```python
from build123d import *
from build123d.topology import SkipClean

# Parameters (mm, degrees)
SKETCH_2_R          = 2
SKETCH_2_R_2        = 11
SKETCH_2_R_3        = 3
SKETCH_2_R_4        = 1.6
EXTRUDE_1_DEPTH     = 10
CUT_EXTRUDE_2_DEPTH = 4


with BuildPart() as part:
    # Эскиз2 → Бобышка-Вытянуть1 (new body)
    with BuildSketch(Plane.XY):
        with BuildLine():
            Line((-25.5006943, 139.9), (-25.5006943, 109.05))
            Line((-25.5006943, 109.05), (-25.5006943, 75.100000001))
            Line((-25.5006943, 75.100000001), (-35.4993057, 75.066643523))
            Line((-35.4993057, 75.066643523), (-35.4993057, 65.066643523))
            Line((-35.4993057, 65.066643523), (-25.5006943, 64.9))
            Line((-25.5006943, 64.9), (-25.5006943, -64.899999999))
            Line((-25.5006943, -64.899999999), (-35.4993057, -64.933356477))
            Line((-35.4993057, -64.933356477), (-35.4993057, -74.933356477))
            Line((-35.4993057, -74.933356477), (-25.5006943, -75.1))
            Line((-25.5006943, -75.1), (-25.5006943, -105.95))
            Line((-25.5006943, -105.95), (-25.5006943, -139.899999999))
            Line((-25.5006943, -139.899999999), (-35.4993057, -139.933356477))
            Line((-35.4993057, -139.933356477), (-35.4993057, -149.933356477))
            Line((-35.4993057, -149.933356477), (-25.5006943, -150.1))
            Line((-25.5006943, -150.1), (-25.5006943, -173.45))
            Line((-25.5006943, -173.45), (-25.5006943, -199.899999999))
            Line((-25.5006943, -199.899999999), (-35.4993057, -199.933356477))
            Line((-35.4993057, -199.933356477), (-35.4993057, -209.933356477))
            Line((-35.4993057, -209.933356477), (-25.5006943, -210.1))
            Line((-25.5006943, -210.1), (-25.5006943, -221))
            Line((-25.5006943, -221), (-17.5006943, -229))
            Line((-17.5006943, -229), (-2.1006943, -229))
            Line((-2.1006943, -229), (-2.067337824, -238.9986114))
            Line((-2.067337824, -238.9986114), (7.932662176, -238.9986114))
            Line((7.932662176, -238.9986114), (8.099305701, -229))
            Line((8.099305701, -229), (35.4993057, -229))
            Line((35.4993057, -229), (35.4993057, -209))
            Line((35.4993057, -209), (33.4993057, -209))
            Line((33.4993057, -209), (33.4993057, -151))
            ThreePointArc((33.4993057, -151), (22.78974844, -0.441666666), (33.4993057, 150.116666668))
            Line((33.4993057, 150.116666668), (33.4993057, 208.116666668))
            Line((33.4993057, 208.116666668), (35.4993057, 208.116666668))
            Line((35.4993057, 208.116666668), (35.4993057, 229))
            Line((35.4993057, 229), (8.099305701, 229))
            Line((8.099305701, 229), (7.932662176, 238.9986114))
            Line((7.932662176, 238.9986114), (-2.067337824, 238.9986114))
            Line((-2.067337824, 238.9986114), (-2.1006943, 229))
            Line((-2.1006943, 229), (-17.5006943, 229))
            Line((-17.5006943, 229), (-25.5006943, 221))
            Line((-25.5006943, 221), (-25.5006943, 210.100000001))
            Line((-25.5006943, 210.100000001), (-35.4993057, 210.066643523))
            Line((-35.4993057, 210.066643523), (-35.4993057, 200.066643523))
            Line((-35.4993057, 200.066643523), (-25.5006943, 199.9))
            Line((-25.5006943, 199.9), (-25.5006943, 176.55))
            Line((-25.5006943, 176.55), (-25.5006943, 150.100000001))
            Line((-25.5006943, 150.100000001), (-35.4993057, 150.066643523))
            Line((-35.4993057, 150.066643523), (-35.4993057, 140.066643523))
            Line((-35.4993057, 140.066643523), (-25.5006943, 139.9))
        make_face()
        with Locations((-18.0006943, -190.5)):
            Circle(SKETCH_2_R, mode=Mode.SUBTRACT)
        with Locations((-18.0006943, -221.5)):
            Circle(SKETCH_2_R, mode=Mode.SUBTRACT)
        with Locations((-18.0006943, 190.5)):
            Circle(SKETCH_2_R, mode=Mode.SUBTRACT)
        with Locations((12.9993057, 221.5)):
            Circle(SKETCH_2_R, mode=Mode.SUBTRACT)
        with Locations((-2.5006943, -206)):
            Circle(SKETCH_2_R_2, mode=Mode.SUBTRACT)
        with Locations((-2.5006943, 206)):
            Circle(SKETCH_2_R_2, mode=Mode.SUBTRACT)
        with Locations((-18.0006943, 221.5)):
            Circle(SKETCH_2_R, mode=Mode.SUBTRACT)
        with Locations((12.9993057, -221.5)):
            Circle(SKETCH_2_R, mode=Mode.SUBTRACT)
        with Locations((12.9993057, -190.5)):
            Circle(SKETCH_2_R, mode=Mode.SUBTRACT)
        with Locations((12.9993057, 190.5)):
            Circle(SKETCH_2_R, mode=Mode.SUBTRACT)
        with Locations((-5.6006943, -153.2)):
            Circle(SKETCH_2_R_3, mode=Mode.SUBTRACT)
        with Locations((-5.6006943, 153.2)):
            Circle(SKETCH_2_R_3, mode=Mode.SUBTRACT)
        with Locations((9.4993057, -139.899999999)):
            Circle(SKETCH_2_R_4, mode=Mode.SUBTRACT)
        with Locations((9.4993057, 139.9)):
            Circle(SKETCH_2_R_4, mode=Mode.SUBTRACT)
    extrude(amount=EXTRUDE_1_DEPTH)

    # Эскиз4 → Вырез-Вытянуть2 (cut)
    with SkipClean():  # the faces are left unmerged after this step: merging them gives an invalid solid
        with BuildSketch(Plane.XY):
            with BuildLine():
                Line((-2.5006943, 217), (35.4993057, 217))
                Line((35.4993057, 217), (35.4993057, 195))
                Line((35.4993057, 195), (-2.5006943, 195))
                ThreePointArc((-2.5006943, 195), (-13.5006943, 206), (-2.5006943, 217))
            make_face()
            with BuildLine():
                Line((-2.5006943, -217), (35.4993057, -217))
                Line((35.4993057, -217), (35.4993057, -195))
                Line((35.4993057, -195), (-2.5006943, -195))
                ThreePointArc((-2.5006943, -195), (-13.5006943, -206), (-2.5006943, -217))
            make_face()
        extrude(amount=CUT_EXTRUDE_2_DEPTH, mode=Mode.SUBTRACT)


solid = part.part
```
Can you work these out from the model? Positions are in its coordinate system, mm. A direction names the side the tool comes from. Give positions to 0.01 mm unless a question says otherwise; leave off trailing zeros. Write each loop counter-clockwise with the first axis right and the second up, starting at its lowest first coordinate (ties: lowest second). Pieces come first, ordered by that corner, then holes. Notation, with made-up numbers: (-5, -23) - (43, -23) arc R29 cw to (43, 2) - close; hole circle Ø1 at (58.25, 20). An arc over 180 degrees is marked (long way). Write item = value, one per line. Start each with the question number.
1. For pin 1 (3 mm diameter, centred on y = -181, z = 3, fed in from -X); pin 2 (1.2 mm diameter, centred on x = 23.5, z = 3, fed in from -Y); pin 3 (2 mm diameter, centred on y = -32.5, z = 4.5, fed in from +X), each with a flat end and sliding along its axis, tell me the tip position at first contact or that it passes through.
2. Imagine slicing it at A-A (z = 5.75). Count the separate pieces of the cut face and the enclosed holes in it, and give its area (3 significant figures).
3. On a 3-axis mill with a long thin cutter (end or side, diameter ignored), from which of +Z, -Z, +X, -X, +Y, -Y can I reach the whole of each face in a straight line? I mean faces 4 (the face through (-25.501, -215, 5)), 5 (the face through (-25.501, 216, 5)), 6 (the face through (3, 238.999, 5)), 7 (the face through (22, 229, 5)), 8 (the face through (-35.499, 205, 5)). Say none if no direction works.
4. Please list where these lines run through material, in increasing order: line 1 (Y direction, x = 21, z = 2); line 2 (Y direction, x = -32, z = 3); line 3 (X direction, y = 190.5, z = 4).
5. Thinking about a two-plate mould opening in Y: for faces 1 (the face through (-25.501, -107, 5)), 2 (the face through (0, 3, 10)), 3 (the face through (22, -229, 5)), which applies, released by +Y, released by -Y, zero draft, split by the parting line, or undercut?
6. Imagine slicing it at B-B (y = 85.5). Please give me the cut outline in (x, z).
7. Imagine slicing it at C-C (y = 35). Please give me the cut outline in (x, z), and give its area (3 significant figures).
Worked answers:
q1.pin_1 = -25.5
q1.pin_2 = -229
q1.pin_3 = 23.3
q2.separate_pieces = 1
q2.enclosed_holes = 14
q2.area = 24,800 mm2
q3.face_4 = +Z, -Z, -X, -Y
q3.face_5 = +Z, -Z, -X, +Y
q3.face_6 = +Z, -Z, +X, -X, +Y
q3.face_7 = +Z, -Z, +X, +Y
q3.face_8 = +Z, -Z, -X, +Y, -Y
q4.line_1 = -229 to -217, -195 to 195, 217 to 229
q4.line_2 = -209.99 to -199.92, -149.99 to -139.92, -74.99 to -64.92, 65.01 to 75.08, 140.01 to 150.08, 200.01 to 210.08
q4.line_3 = -25.5 to -20, -16 to 11, 15 to 33.5
q5.face_1 = undercut
q5.face_2 = zero draft
q5.face_3 = released by -Y
q6.outline = (-25.5, 0) - (26.27, 0) - (26.27, 10) - (-25.5, 10) - close
q7.outline = (-25.5, 0) - (23.38, 0) - (23.38, 10) - (-25.5, 10) - close
q7.area = 489 mm2
